Autodesk Inventor part; units mm, degrees
ref_plane "YZ Plane" through (0, 0, 0) normal (1, 0, 0) x (0, 1, 0)
ref_plane "XZ Plane" through (0, 0, 0) normal (0, 1, 0) x (-1, 0, 0)
ref_plane "XY Plane" through (0, 0, 0) normal (0, 0, 1) x (1, 0, 0)
ref_plane "Work Plane1" through (0, 0, -5) normal (0, 0, 1) x (1, 0, 0)
sketch "Sketch1" plane through (0, 0, -5) normal (0, 0, 1) x (1, 0, 0)
  line L0 (-45, 22) -> (22, 22)
  line L1 (22, 22) -> (22, -22)
  line L2 (22, -22) -> (-45, -22)
  line L3 (-45, -28) -> (-45, -22)
  line L4 (-30, -28) -> (-45, -28)
  line L5 (-30, -28) -> (-28, -30)
  line L6 (-28, -30) -> (28, -30)
  line L7 (28, -30) -> (30, -28)
  line L8 (30, -28) -> (30, 28)
  line L9 (30, 28) -> (28, 30)
  line L10 (28, 30) -> (-28, 30)
  line L11 (-28, 30) -> (-30, 28)
  line L12 (-30, 28) -> (-45, 28)
  line L13 (-45, 22) -> (-45, 28)
  circle A0 centre (25, 25) radius 1.95
  circle A1 centre (25, 0) radius 1.95
  circle A2 centre (0, 25) radius 1.95
  circle A3 centre (-25, -25) radius 1.95
  circle A4 centre (25, -25) radius 1.95
  circle A5 centre (-25, 25) radius 1.95
  circle A6 centre (0, -25) radius 1.95
  line L14 (-30, 28) -> (-30, -28)
  line L15 (22, 22) -> (-22, 22)
  line L16 (-22, 22) -> (-22, -22)
  line L17 (-22, -22) -> (22, -22)
  line L18 (22, -22) -> (22, 22)
  point P0 (0, 0)
  dimension "d0" = 44
  dimension "d1" = 44
extrude "Extrusion1" add sketch "Sketch1" along normal blind 5 contours L0 L14 L11 L10 L9 L8 L7 L6 L5 L2 L1 | L16 L2 L14 L0
properties part number "cellSTORM_v5_cellphonespacer"
Verification items for the finished model (mm, model axes). A direction names the side the tool comes from. Coordinates: 2 decimals unless noted, no trailing zeros. Loops run counter-clockwise (first coordinate to the right, second up) from the corner with the lowest first, then second, coordinate; pieces in that order, holes last. Notation, with made-up numbers: (-40, 80) - (-24, 80) arc R18 ccw to (-24, 111) - close; hole circle Ø1 at (10.5, -27.75). An arc over 180 degrees is marked (long way). Put each result on its own line as item: value.
Item 1: Section check B-B (x = 25). Enter the section's corners in (y, z), then the cut area to 4 significant figures.
Conclusion:
outline: (-30, -5) - (-26.95, -5) - (-26.95, 0) - (-30, 0) - close; (-23.05, -5) - (-1.95, -5) - (-1.95, 0) - (-23.05, 0) - close; (1.95, -5) - (23.05, -5) - (23.05, 0) - (1.95, 0) - close; (26.95, -5) - (30, -5) - (30, 0) - (26.95, 0) - close
area: 241.5 mm2
Item 2: Scan lines: line 1 along Y through (x, z) = (0, -1.5); line 2 along Y through (x, z) = (15, -2.85); line 3 along Y through (x, z) = (25, -4.65). Record each from-to range of solid material in increasing order.
Conclusion:
line 1: y = -30 to -26.95, -23.05 to -22, 22 to 23.05, 26.95 to 30
line 2: y = -30 to -22, 22 to 30
line 3: y = -30 to -26.95, -23.05 to -1.95, 1.95 to 23.05, 26.95 to 30
Item 3: Draft check along X on faces 1 (the face through (-0.1, 22.4, 0)), 2 (the face through (-30, 0, -3)), 3 (the face through (24.746, -26.933, -2.535)), 4 (the face through (22, 0, -3)). Enter one of: pulls with the +X half, pulls with the -X half, needs draft (parallel to the pull), parting line crosses it, or undercut.
Conclusion:
face 1: needs draft
face 2: pulls with the -X half
face 3: undercut
face 4: undercut
Item 4: Section check C-C (z = -1.65). Give the number of separate pieces and of enclosed holes in the cut face, then the cut area to 3 significant figures.
Conclusion:
separate pieces: 1
enclosed holes: 8
area: 1,570 mm2
Item 5: Set-up check for faces 5 (the face through (-22, 0, -3)), 6 (the face through (29, 29, -3)): record each of +Z, -Z, +X, -X, +Y, -Y from which the full face is reachable in a straight line by a thin tool's end or side.
Conclusion:
face 5: +Z, -Z
face 6: +Z, -Z, +X, +Y
Item 6: Section check A-A (y = 0). Enter the section's corners in (x, z), then the cut area to 3 significant figures.
Conclusion:
outline: (-30, -5) - (-22, -5) - (-22, 0) - (-30, 0) - close; (22, -5) - (23.05, -5) - (23.05, 0) - (22, 0) - close; (26.95, -5) - (30, -5) - (30, 0) - (26.95, 0) - close
area: 60.5 mm2
